Check sheet for the modelled part. Datum: model origin and axes. Units: mm. A direction names the side the tool comes from. Coordinates: 2 decimals unless noted, no trailing zeros. Write each loop counter-clockwise with the first axis right and the second up, starting at its lowest first coordinate (ties: lowest second). Pieces come first, ordered by that corner, then holes. Notation, with made-up numbers: (84, 77) -> (129, 77) arc R28 ccw to (129, 105) -> close; hole circle Ø2 at (22.25, 25.25). An arc over 180 degrees is marked (long way). One line per item, written item: value. Start each with the question number.
1) Sectioned sample at A-A on y = -3.5. Enter the section's corners in (x, z) (3 decimals), plus the area to 3 significant figures.
2) Set-up check for faces 1 (the cylindrical face through (-14.48, 0.02, 0.68)), 2 (the cylindrical face through (4.92, 0.021, 10.247)), 3 (the cylindrical face through (3.24, 0.02, -12.93)): record each of +Z, -Z, +X, -X, +Y, -Y from which the full face is reachable in a straight line by a thin tool's end or side.
3) Sectioned sample at B-B on x = 24. Enter the section's corners in (y, z), plus the area to 3 significant figures.
4) Sectioned sample at C-C on y = 0.75. Give the number of separate pieces and of enclosed holes in the cut face, plus the area to 3 significant figures.
5) Scan lines: line 1 along X through (y, z) = (0.25, 1); line 2 along Z through (x, y) = (30, -0.5); line 3 along X through (y, z) = (0.5, 12.75). Record each from-to range of solid material in increasing order. Write a range as [from, to].
6) Draft check along Z on faces 4 (the cylindrical face through (-7.17, 0.02, 10.24)), 5 (the cylindrical face through (-1.112, 0.021, -12.322)), 6 (the flat face through (7, -5.5, 3)), 7 (the cylindrical face through (6.346, 0.021, 10.884)). Enter one of: +Z half, -Z half, draft (parallel to the pull), parting line (faces both ways), or undercut.
7) Gauge pin test, flat ends, axial feed: P1, Ø8.5, axis at x = 19, z = 1, coming from the -Y side; P2, Ø1.5, axis at x = 22, y = 0, coming from the -Z side; P3, Ø12, axis at x = 23, z = -9.5, coming from the -Y side; P4, Ø1.8, axis at x = 29.88, z = -0.23, coming from the +Y side. Record the tip position at first contact, or that the pin passes through.
```python
from build123d import *

# Parameters (mm, degrees)
SKETCH1_R           = 1.5
BOSS_EXTRUDE1_DEPTH = 1.5
BOSS_EXTRUDE2_DEPTH = 4


with BuildPart() as part:
    # Sketch1 → Boss-Extrude1 (new body, symmetric)
    with BuildSketch(Plane(origin=(0, 0, 0), x_dir=(1, 0, 0), z_dir=(0, 1, 0))):
        with BuildLine():
            Line((11.067960149, -3.770386358), (29.879975659, -3.770386358))
            ThreePointArc((29.879975659, -3.770386358), (33.879975659, 0.229613642), (29.879975659, 4.229613642))
            Line((29.879975659, 4.229613642), (11.067960149, 4.229613642))
            ThreePointArc((11.067960149, 4.229613642), (11.847346546, 4.817815376), (12.508067649, 5.536753523))
            ThreePointArc((12.508067649, 5.536753523), (12.391713822, 5.826358841), (12.269206518, 6.113415305))
            ThreePointArc((12.269206518, 6.113415305), (10.921594192, 6.123653667), (9.613413173, 5.799884882))
            ThreePointArc((9.613413173, 5.799884882), (9.35260436, 6.275988642), (9.070690816, 6.73990758))
            ThreePointArc((9.070690816, 6.73990758), (10.005173318, 7.710941183), (10.670112799, 8.883126872))
            ThreePointArc((10.670112799, 8.883126872), (10.482768261, 9.132749542), (10.290139612, 9.378317571))
            ThreePointArc((10.290139612, 9.378317571), (8.985796179, 9.039419334), (7.805987876, 8.38810054))
            ThreePointArc((7.805987876, 8.38810054), (7.430841187, 8.780479171), (7.038462557, 9.155625859))
            ThreePointArc((7.038462557, 9.155625859), (7.68978135, 10.335434163), (8.028679587, 11.639777595))
            ThreePointArc((8.028679587, 11.639777595), (7.783111558, 11.832406244), (7.533488888, 12.019750783))
            ThreePointArc((7.533488888, 12.019750783), (6.361303199, 11.354811301), (5.390269597, 10.420328799))
            ThreePointArc((5.390269597, 10.420328799), (4.926350659, 10.702242344), (4.450246898, 10.963051157))
            ThreePointArc((4.450246898, 10.963051157), (4.774015684, 12.271232176), (4.763777322, 13.618844501))
            ThreePointArc((4.763777322, 13.618844501), (4.476720857, 13.741351805), (4.187115539, 13.857705633))
            ThreePointArc((4.187115539, 13.857705633), (3.22697011, 12.912039434), (2.530885544, 11.758076661))
            ThreePointArc((2.530885544, 11.758076661), (2.009809666, 11.910313178), (1.48242646, 12.039010426))
            ThreePointArc((1.48242646, 12.039010426), (1.45658093, 13.386413785), (1.097903696, 14.685457451))
            ThreePointArc((1.097903696, 14.685457451), (0.78892122, 14.72949474), (0.479069377, 14.766928535))
            ThreePointArc((0.479069377, 14.766928535), (-0.203603467, 13.604981207), (-0.577301983, 12.31017882))
            ThreePointArc((-0.577301983, 12.31017882), (-1.120024341, 12.322363642), (-1.662746699, 12.31017882))
            ThreePointArc((-1.662746699, 12.31017882), (-2.036445216, 13.604981207), (-2.71911806, 14.766928535))
            ThreePointArc((-2.71911806, 14.766928535), (-3.028969902, 14.72949474), (-3.337952378, 14.685457451))
            ThreePointArc((-3.337952378, 14.685457451), (-3.696629612, 13.386413785), (-3.722475143, 12.039010426))
            ThreePointArc((-3.722475143, 12.039010426), (-4.249858349, 11.910313178), (-4.770934227, 11.758076661))
            ThreePointArc((-4.770934227, 11.758076661), (-5.467018792, 12.912039434), (-6.427164221, 13.857705633))
            ThreePointArc((-6.427164221, 13.857705633), (-6.71676954, 13.741351805), (-7.003826004, 13.618844501))
            ThreePointArc((-7.003826004, 13.618844501), (-7.014064366, 12.271232176), (-6.690295581, 10.963051157))
            ThreePointArc((-6.690295581, 10.963051157), (-7.166399341, 10.702242344), (-7.630318279, 10.420328799))
            ThreePointArc((-7.630318279, 10.420328799), (-8.601351881, 11.354811301), (-9.773537571, 12.019750783))
            ThreePointArc((-9.773537571, 12.019750783), (-10.02316024, 11.832406244), (-10.26872827, 11.639777595))
            ThreePointArc((-10.26872827, 11.639777595), (-9.929830033, 10.335434163), (-9.278511239, 9.155625859))
            ThreePointArc((-9.278511239, 9.155625859), (-9.670889869, 8.780479171), (-10.046036558, 8.38810054))
            ThreePointArc((-10.046036558, 8.38810054), (-11.225844862, 9.039419334), (-12.530188294, 9.378317571))
            ThreePointArc((-12.530188294, 9.378317571), (-12.722816943, 9.132749542), (-12.910161481, 8.883126872))
            ThreePointArc((-12.910161481, 8.883126872), (-12.245222, 7.710941183), (-11.310739498, 6.73990758))
            ThreePointArc((-11.310739498, 6.73990758), (-11.592653043, 6.275988642), (-11.853461856, 5.799884882))
            ThreePointArc((-11.853461856, 5.799884882), (-13.161642874, 6.123653667), (-14.5092552, 6.113415305))
            ThreePointArc((-14.5092552, 6.113415305), (-14.631762504, 5.826358841), (-14.748116331, 5.536753523))
            ThreePointArc((-14.748116331, 5.536753523), (-13.802450133, 4.576608094), (-12.64848736, 3.880523528))
            ThreePointArc((-12.64848736, 3.880523528), (-12.800723877, 3.35944765), (-12.929421125, 2.832064444))
            ThreePointArc((-12.929421125, 2.832064444), (-14.276824484, 2.806218913), (-15.57586815, 2.44754168))
            ThreePointArc((-15.57586815, 2.44754168), (-15.619905439, 2.138559204), (-15.657339233, 1.828707361))
            ThreePointArc((-15.657339233, 1.828707361), (-14.495391906, 1.146034517), (-13.200589518, 0.772336))
            ThreePointArc((-13.200589518, 0.772336), (-13.212774341, 0.229613642), (-13.200589518, -0.313108715))
            ThreePointArc((-13.200589518, -0.313108715), (-14.495391906, -0.686807232), (-15.657339233, -1.369480076))
            ThreePointArc((-15.657339233, -1.369480076), (-15.619905439, -1.679331919), (-15.57586815, -1.988314395))
            ThreePointArc((-15.57586815, -1.988314395), (-14.276824484, -2.346991628), (-12.929421125, -2.372837159))
            ThreePointArc((-12.929421125, -2.372837159), (-12.800723877, -2.900220365), (-12.64848736, -3.421296243))
            ThreePointArc((-12.64848736, -3.421296243), (-13.802450133, -4.117380809), (-14.748116331, -5.077526238))
            ThreePointArc((-14.748116331, -5.077526238), (-14.631762504, -5.367131556), (-14.5092552, -5.65418802))
            ThreePointArc((-14.5092552, -5.65418802), (-13.161642874, -5.664426382), (-11.853461856, -5.340657597))
            ThreePointArc((-11.853461856, -5.340657597), (-11.592653043, -5.816761358), (-11.310739498, -6.280680295))
            ThreePointArc((-11.310739498, -6.280680295), (-12.245222, -7.251713898), (-12.910161481, -8.423899587))
            ThreePointArc((-12.910161481, -8.423899587), (-12.722816943, -8.673522257), (-12.530188294, -8.919090286))
            ThreePointArc((-12.530188294, -8.919090286), (-11.225844862, -8.580192049), (-10.046036558, -7.928873256))
            ThreePointArc((-10.046036558, -7.928873256), (-9.670889869, -8.321251886), (-9.278511239, -8.696398575))
            ThreePointArc((-9.278511239, -8.696398575), (-9.929830033, -9.876206878), (-10.26872827, -11.18055031))
            ThreePointArc((-10.26872827, -11.18055031), (-10.02316024, -11.373178959), (-9.773537571, -11.560523498))
            ThreePointArc((-9.773537571, -11.560523498), (-8.601351881, -10.895584017), (-7.630318279, -9.961101514))
            ThreePointArc((-7.630318279, -9.961101514), (-7.166399341, -10.243015059), (-6.690295581, -10.503823872))
            ThreePointArc((-6.690295581, -10.503823872), (-7.014064366, -11.812004891), (-7.003826004, -13.159617217))
            ThreePointArc((-7.003826004, -13.159617217), (-6.71676954, -13.282124521), (-6.427164222, -13.398478348))
            ThreePointArc((-6.427164222, -13.398478348), (-5.467018793, -12.452812149), (-4.770934227, -11.298849376))
            ThreePointArc((-4.770934227, -11.298849376), (-4.249858349, -11.451085894), (-3.722475143, -11.579783141))
            ThreePointArc((-3.722475143, -11.579783141), (-3.696629612, -12.9271865), (-3.337952379, -14.226230166))
            ThreePointArc((-3.337952379, -14.226230166), (-3.028969902, -14.270267455), (-2.71911806, -14.30770125))
            ThreePointArc((-2.71911806, -14.30770125), (-2.036445216, -13.145753923), (-1.662746699, -11.850951535))
            ThreePointArc((-1.662746699, -11.850951535), (-1.120024341, -11.863136358), (-0.577301983, -11.850951535))
            ThreePointArc((-0.577301983, -11.850951535), (-0.203603467, -13.145753923), (0.479069377, -14.30770125))
            ThreePointArc((0.479069377, -14.30770125), (0.78892122, -14.270267455), (1.097903696, -14.226230166))
            ThreePointArc((1.097903696, -14.226230166), (1.45658093, -12.9271865), (1.48242646, -11.579783141))
            ThreePointArc((1.48242646, -11.579783141), (2.009809666, -11.451085893), (2.530885544, -11.298849376))
            ThreePointArc((2.530885544, -11.298849376), (3.22697011, -12.452812149), (4.187115539, -13.398478348))
            ThreePointArc((4.187115539, -13.398478348), (4.476720857, -13.282124521), (4.763777322, -13.159617216))
            ThreePointArc((4.763777322, -13.159617216), (4.774015684, -11.812004891), (4.450246898, -10.503823872))
            ThreePointArc((4.450246898, -10.503823872), (4.926350659, -10.243015059), (5.390269597, -9.961101514))
            ThreePointArc((5.390269597, -9.961101514), (6.361303199, -10.895584017), (7.533488888, -11.560523498))
            ThreePointArc((7.533488888, -11.560523498), (7.783111558, -11.373178959), (8.028679587, -11.18055031))
            ThreePointArc((8.028679587, -11.18055031), (7.68978135, -9.876206878), (7.038462557, -8.696398575))
            ThreePointArc((7.038462557, -8.696398575), (7.430841187, -8.321251886), (7.805987876, -7.928873256))
            ThreePointArc((7.805987876, -7.928873256), (8.985796179, -8.580192049), (10.290139612, -8.919090286))
            ThreePointArc((10.290139612, -8.919090286), (10.482768261, -8.673522257), (10.670112799, -8.423899587))
            ThreePointArc((10.670112799, -8.423899587), (10.005173318, -7.251713898), (9.070690816, -6.280680295))
            ThreePointArc((9.070690816, -6.280680295), (9.35260436, -5.816761358), (9.613413173, -5.340657597))
            ThreePointArc((9.613413173, -5.340657597), (10.921594192, -5.664426382), (12.269206518, -5.65418802))
            ThreePointArc((12.269206518, -5.65418802), (12.391713822, -5.367131556), (12.508067649, -5.077526238))
            ThreePointArc((12.508067649, -5.077526238), (11.847346546, -4.358588091), (11.067960149, -3.770386358))
        make_face()
        with Locations((29.879975659, 0.229613642)):
            Circle(SKETCH1_R, mode=Mode.SUBTRACT)
        with Locations((-1.120024341, 0.229613642)):
            Circle(SKETCH1_R, mode=Mode.SUBTRACT)
    extrude(amount=BOSS_EXTRUDE1_DEPTH, both=True)

    # Sketch2 → Boss-Extrude2 (add)
    with BuildSketch(Plane.XZ.offset(1.5)):
        with BuildLine():
            Line((-0.313290616, 4.715007748), (15.495042643, 3.3195926))
            ThreePointArc((15.495042643, 3.3195926), (18.969975659, -0.229613642), (15.495042643, -3.778819884))
            Line((15.495042643, -3.778819884), (-0.313290616, -5.174235033))
            ThreePointArc((-0.313290616, -5.174235033), (-6.130024341, -0.229613642), (-0.313290616, 4.715007748))
        make_face()
        with BuildLine():
            Line((-0.505153828, 3.22611121), (15.419975659, 1.820386358))
            ThreePointArc((15.419975659, 1.820386358), (17.469975659, -0.229613642), (15.419975659, -2.279613642))
            Line((15.419975659, -2.279613642), (-0.505153828, -3.685338494))
            ThreePointArc((-0.505153828, -3.685338494), (-4.630024341, -0.229613642), (-0.505153828, 3.22611121))
        make_face(mode=Mode.SUBTRACT)
    extrude(amount=BOSS_EXTRUDE2_DEPTH)


solid = part.part
```
Answers:
1. outline: (-0.313, -5.174) -> (15.495, -3.779) arc R3.55 ccw to (15.495, 3.32) -> (-0.313, 4.715) arc R5.01 ccw (long way) to start; hole (-0.505, -3.685) -> (15.42, -2.28) arc R2.05 ccw to (15.42, 1.82) -> (-0.505, 3.226) arc R3.51 ccw (long way) to start
1. area: 83.1 mm2
2. face 1: -X, +Y, -Y
2. face 2: +Y, -Y
2. face 3: -Z, +Y, -Y
3. outline: (-1.5, -4.23) -> (1.5, -4.23) -> (1.5, 3.77) -> (-1.5, 3.77) -> close
3. area: 24.0 mm2
4. separate pieces: 1
4. enclosed holes: 2
4. area: 712 mm2
5. line 1: x = [-15.11, -1.98], [-0.26, 29.02], [30.74, 33.69]
5. line 2: z = [-4.23, -1.72], [1.27, 3.77]
5. line 3: x = [-7.04, -5.72], [-3.72, -1.88], [-0.36, 1.48], [3.48, 4.8]
6. face 4: undercut
6. face 5: -Z half
6. face 6: draft
6. face 7: +Z half
7. P1: stops at y = -5.5
7. P2: stops at z = -4.23
7. P3: stops at y = -1.5
7. P4: passes through
